Can you work these out from the drawing? Everything is in mm from the part's minimum corner. A direction names the side the tool comes from. Give positions to 0.01 mm unless a question says otherwise; leave off trailing zeros. Loops run counter-clockwise (first coordinate to the right, second up) from the corner with the lowest first, then second, coordinate; pieces in that order, holes last. Notation, with made-up numbers: (49.25, 29) - (62.25, 29) arc R5 cw to (62.25, 34) - close; hole circle Ø7 at (57, 44.25). An arc over 180 degrees is marked (long way). One line per item, written item: value. Start each with the question number.
Q1. I want a section at C-C (x = 11). Please give me the cut outline in (y, z).
Q2. For the marked faces 1 and 2, which set-ups out of +Z, -Z, +X, -X, +Y, -Y let a thin tool reach every point of the face, with its end or its side?
Q3. I want a section at B-B (y = 2.75). Please give me the cut outline in (x, z).
Q4. I want a section at A-A (z = 5.25). Please give me the cut outline in (x, y), then the cut area to 3 significant figures.
Q5. If we mould it in two halves opening along X, with no side actions, what happens to the marked faces 3, 4, 5 and 6? For each: released by +X, released by -X, zero draft, split by the parting line, or undercut.
Q6. I want a section at D-D (z = 1). Please give me the cut outline in (x, y).
Q7. If I drill on line 1 (X direction, y = 2, z = 7.25); line 2 (Z direction, x = 4, y = 1.25); line 3 (X direction, y = 5, z = 2), over which ranges is the centre line in solid material (lowest first)? Write a range as from..to.
Q8. I'm going to push flat-ended pins straight in: P1, Ø3, axis at x = 20.5, y = 3.5, coming from the +Z side; P2, Ø1, axis at y = 2, z = 1.5, coming from the -X side. Where does each tip first touch, or does it pass through?
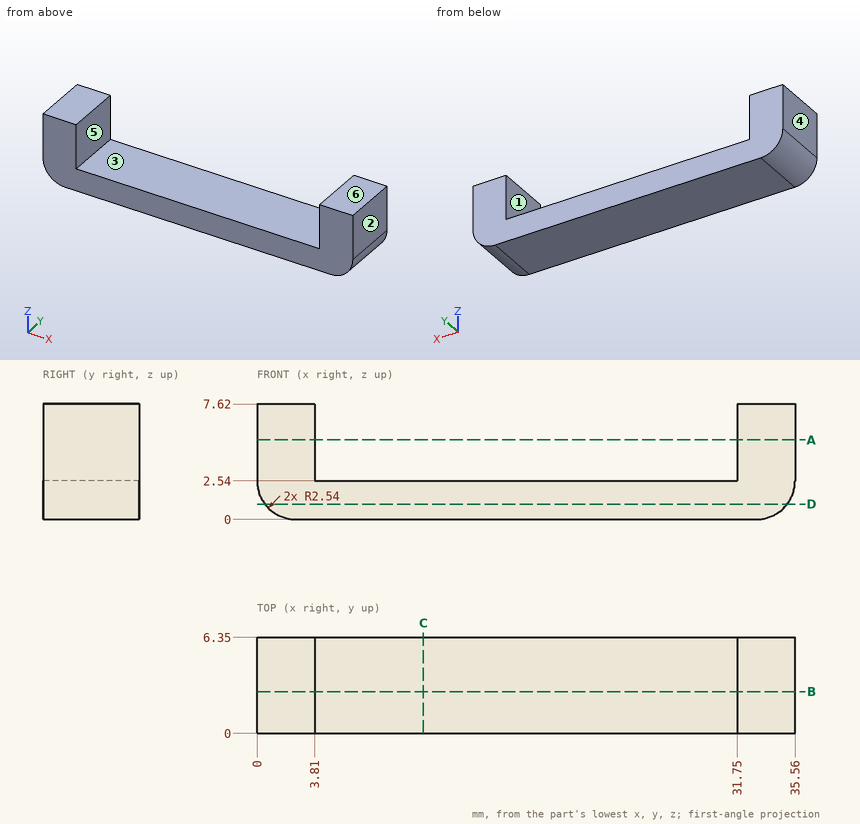
Worked answers:
1. outline: (0, 0) - (6.35, 0) - (6.35, 2.54) - (0, 2.54) - close
2. face 1: +Z, +Y, -Y
2. face 2: +Z, -Z, +X, +Y, -Y
3. outline: (0, 2.54) arc R2.54 ccw to (2.54, 0) - (33.02, 0) arc R2.54 ccw to (35.56, 2.54) - (35.56, 7.62) - (31.75, 7.62) - (31.75, 2.54) - (3.81, 2.54) - (3.81, 7.62) - (0, 7.62) - close
4. outline: (0, 0) - (3.81, 0) - (3.81, 6.35) - (0, 6.35) - close; (31.75, 0) - (35.56, 0) - (35.56, 6.35) - (31.75, 6.35) - close
4. area: 48.4 mm²
5. face 3: undercut
5. face 4: released by -X
5. face 5: undercut
5. face 6: zero draft
6. outline: (0.52, 0) - (35.04, 0) - (35.04, 6.35) - (0.52, 6.35) - close
7. line 1: x = 0..3.81, 31.75..35.56
7. line 2: z = 0..2.54
7. line 3: x = 0.06..35.5
8. P1: stops at z = 2.54
8. P2: stops at x = 0.06
